Check sheet for the modelled part. Datum: model origin and axes. Units: mm. Face numbers are marked on the shaded views. A direction names the side the tool comes from. Give positions to 0.01 mm unless a question says otherwise; leave off trailing zeros. Write each loop counter-clockwise with the first axis right and the second up, starting at its lowest first coordinate (ties: lowest second). Pieces come first, ordered by that corner, then holes. Notation, with made-up numbers: (-7, 0.25) - (42, 0.25) arc R27 cw to (42, 34.25) - close; hole circle Ø4 at (-5, 50). An arc over 180 degrees is marked (long way). Return JSON: item names as keys, results as strings. Group by question number.
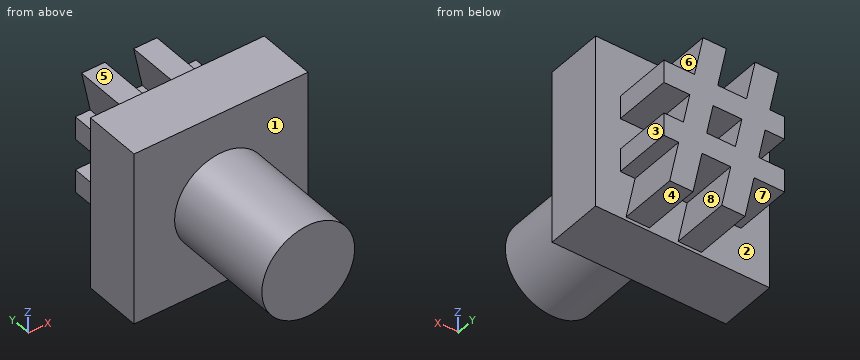
```python
from build123d import *

# Parameters (mm, degrees)
SKETCH1_W           = 15
SKETCH1_H           = 15
BOSS_EXTRUDE1_DEPTH = 5
BOSS_EXTRUDE2_DEPTH = 5
SKETCH3_R           = 4
BOSS_EXTRUDE3_DEPTH = 10


with BuildPart() as part:
    # Sketch1 → Boss-Extrude1 (new body)
    with BuildSketch(Plane(origin=(0, 0, 0), x_dir=(1, 0, 0), z_dir=(0, 1, 0))):
        Rectangle(SKETCH1_W, SKETCH1_H)
    extrude(amount=BOSS_EXTRUDE1_DEPTH)

    # Sketch2 → Boss-Extrude2 (add)
    with BuildSketch(Plane(origin=(0, 5, 0), x_dir=(1, 0, 0), z_dir=(0, 1, 0))):
        Polygon((-3.754056884, -3.202967132), (-5.03009855, -3.202967132), (-5.03009855, -1.228608158), (-3.35021073, -1.228608158), (-2.797726755, 1.463699535), (-5.03009855, 1.463699535), (-5.03009855, 3.438058509), (-2.393880602, 3.438058509), (-1.61984214, 7.207289278), (0.38817068, 7.207289278), (-0.385867781, 3.438058509), (2.093298886, 3.438058509), (2.867337347, 7.207289278), (4.875350168, 7.207289278), (4.101311706, 3.438058509), (5.38015786, 3.438058509), (5.38015786, 1.463699535), (3.697465552, 1.463699535), (3.144981578, -1.228608158), (5.38015786, -1.228608158), (5.38015786, -3.202967132), (2.741135424, -3.202967132), (2.003555296, -6.792710722), (-0.004457525, -6.792710722), (0.733122604, -3.202967132), (-1.746044063, -3.202967132), (-2.483624191, -6.792710722), (-4.491637012, -6.792710722), align=None)
        Polygon((-0.789713935, 1.463699535), (-1.342197909, -1.228608158), (1.136968757, -1.228608158), (1.689452732, 1.463699535), align=None, mode=Mode.SUBTRACT)
    extrude(amount=BOSS_EXTRUDE2_DEPTH)

    # Sketch3 → Boss-Extrude3 (add)
    with BuildSketch(Plane.XZ):
        with Locations(Location((0, 0, 0), (0, 0, 270))):
            Circle(SKETCH3_R)
    extrude(amount=BOSS_EXTRUDE3_DEPTH)


solid = part.part
```
Item 1: Section check B-B on z = 0.5. Record the cut outline in (x, y).
Item 2: Material ranges on line 1 along Z through (x, y) = (-0.5, 6); line 2 along Y through (x, z) = (3, 5.5); line 3 along Y through (x, z) = (1, 0), recorded low to high. Write a range as from..to.
Item 3: Depth check by flat-ended pin: pin 1 (2 mm diameter, centred on y = 8.5, z = -2.5, fed in from +X); pin 2 (5 mm diameter, centred on x = -0.5, y = -7.5, fed in from -Z); pin 3 (2 mm diameter, centred on x = -4, y = 8.5, fed in from +Z). Enter the tip coordinate at first touch or a pass-through.
Item 4: Section check C-C on x = 6. Record the cut outline in (y, z), plus the area to 3 significant figures.
Item 5: Mould release check, pull along X, two halves, no side actions. Record for the marked faces 1, 2 and 3: +X half, -X half, draft (parallel to the pull), parting line (faces both ways), or undercut.
Item 6: Section check D-D on y = -7. Record the cut outline in (x, z), plus the area to 3 significant figures.
Item 7: Access from +Z, -Z, +X, -X, +Y, -Y to the whole of each face (thin tool, end or side, straight path). Record for the marked faces 4, 5, 6, 7 and 8.
Reply:
{
 "1": {"outline": "(-7.5, 0) - (-3.97, 0) - (-3.97, -10) - (3.97, -10) - (3.97, 0) - (7.5, 0) - (7.5, 5) - (3.29, 5) - (3.29, 10) - (1.29, 10) - (1.29, 5) - (-1.19, 5) - (-1.19, 10) - (-3.2, 10) - (-3.2, 5) - (-7.5, 5) - close"},
 "2": {"line 1": "-7.21..-1.46, 1.23..3.2", "line 2": "0..5", "line 3": "-10..5"},
 "3": {"pin 1": "x = 5.38", "pin 2": "z = -4", "pin 3": "z = 6.79"},
 "4": {"outline": "(0, -7.5) - (5, -7.5) - (5, 7.5) - (0, 7.5) - close", "area": "75.0 mm²"},
 "5": {"face 1": "draft", "face 2": "undercut", "face 3": "+X half"},
 "6": {"outline": "circle Ø8 at (0, 0)", "area": "50.3 mm²"},
 "7": {"face 4": "-Z, +X, -X, +Y", "face 5": "+Z, +X, -X, +Y", "face 6": "+Z, +X, +Y", "face 7": "-Z, -X, +Y", "face 8": "+Y"}
}
